from build123d import *

# Parameters (mm, degrees)
F0_W      = 56
F0_H      = 56
F0_W_2    = 8
F0_H_2    = 8
F1_DEPTH  = 10
F3_START  = -6
F3_DEPTH  = 4
F4_D      = 3.3
F4_DEPTH  = 10
F4_TIP    = 0.9914200214
F5_D      = 5.8
F5_DEPTH  = 1.5
F5_TIP    = 1.7424957952
F7_START  = -6
F7_DEPTH  = 4
F8_D      = 5.8
F8_DEPTH  = 1.5
F8_TIP    = 1.7424957952
F9_D      = 3.3
F9_DEPTH  = 10
F9_START  = 2.2510758
F9_TIP    = 0.9914200214
F11_START = -6
F11_DEPTH = 4
F12_D     = 3.3
F12_DEPTH = 10
F12_TIP   = 0.9914200214
F13_D     = 5.8
F13_DEPTH = 1.5
F13_TIP   = 1.7424957952
F15_START = -6
F15_DEPTH = 4
F16_D     = 5.8
F16_DEPTH = 1.5
F16_TIP   = 1.7424957952
F17_D     = 3.3
F17_DEPTH = 10
F17_START = 2.2510758
F17_TIP   = 0.9914200214
F18_SIZE  = 1
F19_D     = 5.1054
F19_DEPTH = 15.81
F19_TIP   = 1.5338169022


with BuildPart() as f1:
    # F0 (on Front) → F1 (new body)
    with BuildSketch(Plane.XZ):
        Rectangle(F0_W, F0_H)
        with BuildLine():
            ThreePointArc((20, -18), (19.4142135624, -19.4142135624), (18, -20))
            Line((18, -20), (6, -20))
            ThreePointArc((6, -20), (4.5857864376, -19.4142135624), (4, -18))
            Line((4, -18), (4, -9.1651513899))
            ThreePointArc((4, -9.1651513899), (0, -10), (-4, -9.1651513899))
            Line((-4, -9.1651513899), (-4, -18))
            ThreePointArc((-4, -18), (-4.5857864376, -19.4142135624), (-6, -20))
            Line((-6, -20), (-18, -20))
            ThreePointArc((-18, -20), (-19.4142135624, -19.4142135624), (-20, -18))
            Line((-20, -18), (-20, -6))
            ThreePointArc((-20, -6), (-19.4142135624, -4.5857864376), (-18, -4))
            Line((-18, -4), (-9.1651513899, -4))
            ThreePointArc((-9.1651513899, -4), (-10, 0), (-9.1651513899, 4))
            Line((-9.1651513899, 4), (-18, 4))
            ThreePointArc((-18, 4), (-19.4142135624, 4.5857864376), (-20, 6))
            Line((-20, 6), (-20, 18))
            ThreePointArc((-20, 18), (-19.4142135624, 19.4142135624), (-18, 20))
            Line((-18, 20), (-6, 20))
            ThreePointArc((-6, 20), (-4.5857864376, 19.4142135624), (-4, 18))
            Line((-4, 18), (-4, 9.1651513899))
            ThreePointArc((-4, 9.1651513899), (0, 10), (4, 9.1651513899))
            Line((4, 9.1651513899), (4, 18))
            ThreePointArc((4, 18), (4.5857864376, 19.4142135624), (6, 20))
            Line((6, 20), (18, 20))
            ThreePointArc((18, 20), (19.4142135624, 19.4142135624), (20, 18))
            Line((20, 18), (20, 6))
            ThreePointArc((20, 6), (19.4142135624, 4.5857864376), (18, 4))
            Line((18, 4), (9.1651513899, 4))
            ThreePointArc((9.1651513899, 4), (9.7890631293, 2.0430964369), (10, 0))
            ThreePointArc((10, 0), (9.7890631293, -2.0430964369), (9.1651513899, -4))
            Line((9.1651513899, -4), (18, -4))
            ThreePointArc((18, -4), (19.4142135624, -4.5857864376), (20, -6))
            Line((20, -6), (20, -18))
        make_face(mode=Mode.SUBTRACT)
        with BuildLine():
            Line((-9.1651513899, 4), (-4, 4))
            Line((-4, 4), (-4, 9.1651513899))
            ThreePointArc((-4, 9.1651513899), (-7.0710678119, 7.0710678119), (-9.1651513899, 4))
        make_face()
        with BuildLine():
            Line((-4, 4), (4, 4))
            Line((4, 4), (4, 9.1651513899))
            ThreePointArc((4, 9.1651513899), (0, 10), (-4, 9.1651513899))
            Line((-4, 9.1651513899), (-4, 4))
        make_face()
        with BuildLine():
            Line((4, 9.1651513899), (4, 4))
            Line((4, 4), (9.1651513899, 4))
            ThreePointArc((9.1651513899, 4), (7.0710678119, 7.0710678119), (4, 9.1651513899))
        make_face()
        with BuildLine():
            Line((4, 4), (4, -4))
            Line((4, -4), (9.1651513899, -4))
            ThreePointArc((9.1651513899, -4), (9.7890631293, -2.0430964369), (10, 0))
            ThreePointArc((10, 0), (9.7890631293, 2.0430964369), (9.1651513899, 4))
            Line((9.1651513899, 4), (4, 4))
        make_face()
        with BuildLine():
            Line((4, -4), (4, -9.1651513899))
            ThreePointArc((4, -9.1651513899), (7.0710678119, -7.0710678119), (9.1651513899, -4))
            Line((9.1651513899, -4), (4, -4))
        make_face()
        with BuildLine():
            ThreePointArc((-4, -9.1651513899), (0, -10), (4, -9.1651513899))
            Line((4, -9.1651513899), (4, -4))
            Line((4, -4), (-4, -4))
            Line((-4, -4), (-4, -9.1651513899))
        make_face()
        with BuildLine():
            ThreePointArc((-9.1651513899, -4), (-7.0710678119, -7.0710678119), (-4, -9.1651513899))
            Line((-4, -9.1651513899), (-4, -4))
            Line((-4, -4), (-9.1651513899, -4))
        make_face()
        with BuildLine():
            Line((-9.1651513899, -4), (-4, -4))
            Line((-4, -4), (-4, 4))
            Line((-4, 4), (-9.1651513899, 4))
            ThreePointArc((-9.1651513899, 4), (-10, 0), (-9.1651513899, -4))
        make_face()
        Rectangle(F0_W_2, F0_H_2)
    extrude(amount=F1_DEPTH)

    # F2 (on face) → F3 (cut)
    with BuildSketch(Plane.YZ.offset(28).offset(F3_START)):
        Polygon((-7.8785498805, 6.7890692829), (-4.9575654752, 5.1516373189), (-2.0790155946, 6.8625680359), (-2.1214501195, 10.2109307171), (-5.0424345248, 11.8483626811), (-7.9209844054, 10.1374319641), align=None)
        Polygon((-7.8785498805, -10.2109307171), (-4.9575654752, -11.8483626811), (-2.0790155946, -10.1374319641), (-2.1214501195, -6.7890692829), (-5.0424345248, -5.1516373189), (-7.9209844054, -6.8625680359), align=None)
    extrude(amount=-F3_DEPTH, mode=Mode.SUBTRACT)

    # F4
    with Locations(Plane.YZ.offset(28)):
        with Locations((-5, -8.5), (-5, 8.5)):
            Hole(F4_D / 2, depth=F4_DEPTH)
            with Locations((0, 0, -(F4_DEPTH + F4_TIP / 2))):  # 118° drill point
                Cone(0, F4_D / 2, F4_TIP, mode=Mode.SUBTRACT)

    # F5
    with Locations(Plane.YZ.offset(28)):
        with Locations((-5, 8.5), (-5, -8.5)):
            Hole(F5_D / 2, depth=F5_DEPTH)
            with Locations((0, 0, -(F5_DEPTH + F5_TIP / 2))):  # 118° drill point
                Cone(0, F5_D / 2, F5_TIP, mode=Mode.SUBTRACT)

    # F6 (on face) → F7 (cut)
    with BuildSketch(Plane(origin=(0, 0, -28), x_dir=(1, 0, 0), z_dir=(0, 0, -1)).offset(F7_START)):
        Polygon((6.8256842194, 7.9), (5.1513684387, 5), (6.8256842194, 2.1), (10.1743157806, 2.1), (11.8486315613, 5), (10.1743157806, 7.9), align=None)
        Polygon((-10.1743157806, 7.9), (-11.8486315613, 5), (-10.1743157806, 2.1), (-6.8256842194, 2.1), (-5.1513684387, 5), (-6.8256842194, 7.9), align=None)
    extrude(amount=-F7_DEPTH, mode=Mode.SUBTRACT)

    # F8
    with Locations(Plane(origin=(0, 0, -28), x_dir=(1, 0, 0), z_dir=(0, 0, -1))):
        with Locations((8.5, 5), (-8.5, 5)):
            Hole(F8_D / 2, depth=F8_DEPTH)
            with Locations((0, 0, -(F8_DEPTH + F8_TIP / 2))):  # 118° drill point
                Cone(0, F8_D / 2, F8_TIP, mode=Mode.SUBTRACT)

    # F9
    # its depths count from where the whole tool has entered the part; down to there all is cleared
    with Locations(Plane(origin=(0, 0, -28), x_dir=(1, 0, 0), z_dir=(0, 0, -1)).offset(-F9_START)):
        with Locations((8.5, 5), (-8.5, 5)):
            Hole(F9_D / 2, depth=F9_DEPTH)
            with Locations((0, 0, -(F9_DEPTH + F9_TIP / 2))):  # 118° drill point
                Cone(0, F9_D / 2, F9_TIP, mode=Mode.SUBTRACT)

    # F10 (on face) → F11 (cut)
    with BuildSketch(Plane(origin=(-28, 0, 0), x_dir=(0, -1, 0), z_dir=(-1, 0, 0)).offset(F11_START)):
        Polygon((7.9, -6.8256842194), (5, -5.1513684387), (2.1, -6.8256842194), (2.1, -10.1743157806), (5, -11.8486315613), (7.9, -10.1743157806), align=None)
        Polygon((7.9, 10.1743157806), (5, 11.8486315613), (2.1, 10.1743157806), (2.1, 6.8256842194), (5, 5.1513684387), (7.9, 6.8256842194), align=None)
    extrude(amount=-F11_DEPTH, mode=Mode.SUBTRACT)

    # F12
    with Locations(Plane(origin=(-28, 0, 0), x_dir=(0, -1, 0), z_dir=(-1, 0, 0))):
        with Locations((5, -8.5), (5, 8.5)):
            Hole(F12_D / 2, depth=F12_DEPTH)
            with Locations((0, 0, -(F12_DEPTH + F12_TIP / 2))):  # 118° drill point
                Cone(0, F12_D / 2, F12_TIP, mode=Mode.SUBTRACT)

    # F13
    with Locations(Plane(origin=(-28, 0, 0), x_dir=(0, -1, 0), z_dir=(-1, 0, 0))):
        with Locations((5, -8.5), (5, 8.5)):
            Hole(F13_D / 2, depth=F13_DEPTH)
            with Locations((0, 0, -(F13_DEPTH + F13_TIP / 2))):  # 118° drill point
                Cone(0, F13_D / 2, F13_TIP, mode=Mode.SUBTRACT)

    # F14 (on face) → F15 (cut)
    with BuildSketch(Plane.XY.offset(28).offset(F15_START)):
        Polygon((-6.8256842194, -7.9), (-5.1513684387, -5), (-6.8256842194, -2.1), (-10.1743157806, -2.1), (-11.8486315613, -5), (-10.1743157806, -7.9), align=None)
        Polygon((6.8256842194, -7.9), (10.1743157806, -7.9), (11.8486315613, -5), (10.1743157806, -2.1), (6.8256842194, -2.1), (5.1513684387, -5), align=None)
    extrude(amount=-F15_DEPTH, mode=Mode.SUBTRACT)

    # F16
    with Locations(Plane.XY.offset(28)):
        with Locations((-8.5, -5), (8.5, -5)):
            Hole(F16_D / 2, depth=F16_DEPTH)
            with Locations((0, 0, -(F16_DEPTH + F16_TIP / 2))):  # 118° drill point
                Cone(0, F16_D / 2, F16_TIP, mode=Mode.SUBTRACT)

    # F17
    # its depths count from where the whole tool has entered the part; down to there all is cleared
    with Locations(Plane.XY.offset(28).offset(-F17_START)):
        with Locations((-8.5, -5), (8.5, -5)):
            Hole(F17_D / 2, depth=F17_DEPTH)
            with Locations((0, 0, -(F17_DEPTH + F17_TIP / 2))):  # 118° drill point
                Cone(0, F17_D / 2, F17_TIP, mode=Mode.SUBTRACT)

    # F18
    f18_edges = [f1.edges().sort_by_distance(p)[0] for p in [
        (28, -5, 28),
        (28, -5, -28),
        (-28, -5, -28),
        (-28, -5, 28),
    ]]
    chamfer(f18_edges, length=F18_SIZE)

    # F19
    with Locations(Plane(origin=(0, 0, 0), x_dir=(1, 0, 0), z_dir=(0, 1, 0))):
        with Locations((0, 0)):
            Hole(F19_D / 2, depth=F19_DEPTH)
            with Locations((0, 0, -(F19_DEPTH + F19_TIP / 2))):  # 118° drill point
                Cone(0, F19_D / 2, F19_TIP, mode=Mode.SUBTRACT)


solid = f1.part
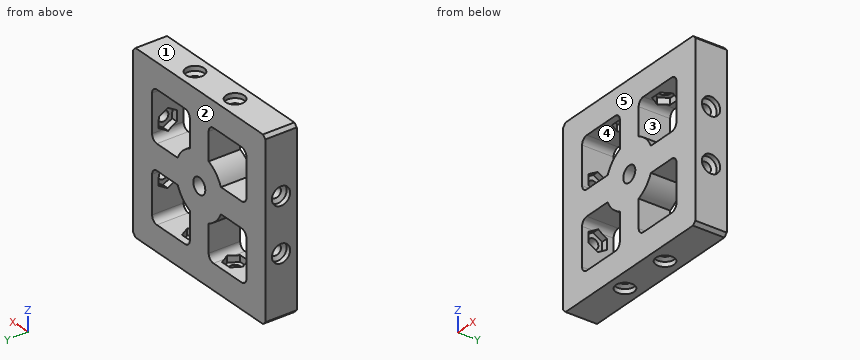
For this review, take the finished solid that the model builds, in its own axes (mm). Face numbers are marked on the shaded views. A direction names the side the tool comes from. Coordinates: 2 decimals unless noted, no trailing zeros. Order: outer loops, then holes, each group sorted by start corner. A loop starts at its lowest first (then second) coordinate and runs counter-clockwise, first axis right, second up. Notation, with made-up numbers: (-27.5, 25) - (26.5, 25) arc R32 ccw to (26.5, 63) - close; hole circle Ø1 at (76, 21). An arc over 180 degrees is marked (long way). Answer as CSV lines item,"result". Start each with the question number.
1) Add section B-B (z = 16.5). State the section outline as (x, y) points, then the cut area to 3 significant figures.
2) To check wall thickness, follow line 1 along X through (y, z) = (-5, 23.3); line 2 along Z through (x, y) = (27, -5). State the ranges of each line that lie inside material, in increasing order. Write a range as [from, to].
3) Add section C-C (x = 23.5). State the section outline as (y, z) points, then the cut area to 3 significant figures.
4) Machinability: for the marked faces 4 and 5, which of the approach directions +Z, -Z, +X, -X, +Y, -Y give a long, thin tool a straight path to every point of the face, cutting with its end or side? Answer none if there is none.
5) Insertion check: P1, Ø2, axis at x = -8.5, y = -5, coming from the -Z side; P2, Ø3.5, axis at x = -8.5, y = -5, coming from the -Z side; P3, Ø1.8, axis at y = -3.5, z = -9.5, coming from the -X side. Each pin has a flat end and moves straight along its axis. Give the tip position at first contact, or say it passes through.
6) Draft analysis for pull direction Z (two halves, no side actions). For the marked faces 1, 2 and 3, state which applies: +Z half, -Z half, draft (parallel to the pull), parting line (faces both ways), or undercut.
7) Add section A-A (x = 0). State the section outline as (y, z) points, then the cut area to 3 significant figures.
8) Add section D-D (y = -4.25). Count the separate pieces of the cut face and the enclosed holes in it, then the cut area to 3 significant figures.
Result:
1,outline,"(-28, -10) - (-20, -10) - (-20, 0) - (-28, 0) - close; (-4, -10) - (4, -10) - (4, 0) - (-4, 0) - close; (20, -10) - (28, -10) - (28, 0) - (20, 0) - close"
1,area,"240 mm^2"
2,line 1,"[-28, -10.15], [-6.85, 6.85], [10.15, 28]"
2,line 2,"[-28, -11.4], [-5.6, 5.6], [11.4, 28]"
3,outline,"(-10, -28) - (0, -28) - (0, 28) - (-10, 28) - close; hole circle Ø3.3 at (-5, -8.5); hole circle Ø3.3 at (-5, 8.5)"
3,area,"543 mm^2"
4,face 4,"+Y, -Y"
4,face 5,"+Z, -Z, +X, -X, -Y"
5,P1,"z = -6.61"
5,P2,"z = -25.81"
5,P3,"x = -26.38"
6,face 1,"+Z half"
6,face 2,"draft"
6,face 3,"undercut"
7,outline,"(-10, -28) - (0, -28) - (0, -2.55) - (-10, -2.55) - close; (-10, 2.55) - (0, 2.55) - (0, 28) - (-10, 28) - close"
7,area,"509 mm^2"
8,separate pieces,"5"
8,enclosed holes,"1"
8,area,"1,890 mm^2"
